```python
from build123d import *

# Parameters (mm, degrees)
REVOLVE_1_ANGLE          = 180
CUT_EXTRUDE_3_DEPTH      = 21.784609691
CUT_EXTRUDE_3_DEPTH_BACK = 21.784609691
SKETCH_5_W               = 8
SKETCH_5_H               = 30
SKETCH_11_R              = 6.6
CUT_EXTRUDE_7_DEPTH      = 18.435595774
SKETCH_12_R              = 9
CUT_EXTRUDE_8_DEPTH      = 2


with BuildPart() as part:
    # 草图1 → 旋转1 (revolve)
    with BuildSketch(Plane(origin=(0, 0, 0), x_dir=(0, 0, -1), z_dir=(1, 0, 0))):
        with BuildLine():
            Line((0, 12), (0, -12))
            ThreePointArc((0, -12), (-12, 0), (0, 12))
        make_face()
    revolve(axis=Axis((0, 12, 0), (0, -1, 0)), revolution_arc=REVOLVE_1_ANGLE)

    # 草图5 → 切除-拉伸3 (cut, two sides: drawn at the far end of the back side and taken through both)
    with BuildSketch(Plane.XY.offset(-CUT_EXTRUDE_3_DEPTH_BACK)):
        with Locations((-8, 0.775192037)):
            Rectangle(SKETCH_5_W, SKETCH_5_H)
    extrude(amount=CUT_EXTRUDE_3_DEPTH + CUT_EXTRUDE_3_DEPTH_BACK, mode=Mode.SUBTRACT)


with BuildPart() as cut_extrude_3_kept_piece:
    # of the separate pieces the step leaves, the one the design keeps (cut_extrude_3_pieces_kept)
    add(part.part.solids().sort_by_distance((0, -12, 0))[0])

    # 草图11 → 切除-拉伸7 (cut, through all)
    with BuildSketch(Plane(origin=(0, 0, 0), x_dir=(0, 0, -1), z_dir=(1, 0, 0))):
        Circle(SKETCH_11_R)
    extrude(amount=-CUT_EXTRUDE_7_DEPTH, mode=Mode.SUBTRACT)

    # 草图12 → 切除-拉伸8 (cut)
    with BuildSketch(Plane(origin=(0, 0, 0), x_dir=(0, 0, -1), z_dir=(1, 0, 0))):
        Circle(SKETCH_12_R)
    extrude(amount=-CUT_EXTRUDE_8_DEPTH, mode=Mode.SUBTRACT)


solid = cut_extrude_3_kept_piece.part
```
CAD build for the part. Positions are in the model's coordinates, mm. A direction names the side the tool comes from. Coordinates: 2 decimals unless noted, no trailing zeros. Write each loop counter-clockwise with the first axis right and the second up, starting at its lowest first coordinate (ties: lowest second). Pieces come first, ordered by that corner, then holes. Notation, with made-up numbers: (53, -3.5) -> (76, -3.5) arc R26 cw to (76, 30.5) -> close; hole circle Ø11 at (59.25, 63). An arc over 180 degrees is marked (long way). Return JSON: item names as keys, results as strings. Group by question number.
Q1. Cut at D-D, the plane x = -1.55. Give the cut face in (y, z).
Q2. Cut at C-C, the plane y = 7. Give the cut face in (x, z), then the cut area to 3 significant figures.
Q3. Drill centre lines: line 1 (Y direction, x = -0.75, z = 5); line 2 (Z direction, x = -3.65, y = 6); line 3 (Z direction, x = -2.7, y = -3). Where is each one in solid material? Low to high.
Q4. Which spindle directions (+Z, -Z, +X, -X, +Y, -Y) get a long thin tool onto all of the face, cutting with end or side? Do faces 3 (the face through (-2, 5, 5)), 4 (the face through (-2.986, 4.461, 4.864)). Say none if no direction does.
Q5. Pull direction Z, two halves, no side cores. Call faces 1 (the face through (-0.986, 8.923, 1.172)), 2 (the face through (-4, 5, 5)): released by +Z, released by -Z, zero draft, split by the parting line, or undercut.
Q6. Cut at A-A, the plane y = 0. Give the cut face in (x, z).
Returned:
{
 "1": {"outline": "circle Ø23.8 at (0, 0); hole circle Ø18 at (0, 0)"},
 "2": {"outline": "(-4, -8.89) arc R9.75 ccw to (0, -9.75) -> (0, -5.66) -> (-2, -5.66) -> (-2, 5.66) -> (0, 5.66) -> (0, 9.75) arc R9.75 ccw to (-4, 8.89) -> close", "area": "53.1 mm2"},
 "3": {"line 1": "y = -10.88 to -7.48, 7.48 to 10.88", "line 2": "z = -9.73 to -2.75, 2.75 to 9.73", "line 3": "z = -11.3 to -5.88, 5.88 to 11.3"},
 "4": {"face 3": "+X", "face 4": "+X, -X"},
 "5": {"face 1": "undercut", "face 2": "zero draft"},
 "6": {"outline": "(-4, -11.31) arc R12 ccw to (0, -12) -> (0, -9) -> (-2, -9) -> (-2, -6.6) -> (-4, -6.6) -> close; (-4, 6.6) -> (-2, 6.6) -> (-2, 9) -> (0, 9) -> (0, 12) arc R12 ccw to (-4, 11.31) -> close"}
}
